from build123d import *

# Parameters (mm, degrees)
ESTRUSIONE_ESTRUSIONE1_DEPTH = 17
SCHIZZO2_W                   = 25
SCHIZZO2_H                   = 30
TAGLIO_ESTRUSIONE1_DEPTH     = 17


with BuildPart() as part:
    # Schizzo1 → Estrusione-Estrusione1 (new body)
    with BuildSketch(Plane.XY):
        with BuildLine():
            Line((0, 0), (85, 0))
            Line((85, 0), (85, 25))
            ThreePointArc((85, 25), (83.753843891, 36.016505892), (80.078350515, 46.47628866))
            Line((80.078350515, 46.47628866), (30, 150))
            Line((30, 150), (0, 150))
            Line((0, 150), (0, 0))
        make_face()
    extrude(amount=ESTRUSIONE_ESTRUSIONE1_DEPTH)

    # Schizzo2 → Taglio-Estrusione1 (cut)
    with BuildSketch(Plane(origin=(0, 0, 0), x_dir=(-1, 0, 0), z_dir=(0, 0, -1))):
        with Locations((-12.5, 15)):
            Rectangle(SCHIZZO2_W, SCHIZZO2_H)
    extrude(amount=-TAGLIO_ESTRUSIONE1_DEPTH, mode=Mode.SUBTRACT)


solid = part.part
Can you work these out from the model? Positions are in its coordinate system, mm. A direction names the side the tool comes from. Give positions to 0.01 mm unless a question says otherwise; leave off trailing zeros. Order: outer loops, then holes, each group sorted by start corner. A loop starts at its lowest first (then second) coordinate and runs counter-clockwise, first axis right, second up. Notation, with made-up numbers: M -5.75,66.5 L 3.25,66.5 A36 cw 3.25,104.5 Z; hole C -16.5,59.5 d2. An arc over 180 degrees is marked long. Use a Markdown table: item, result. Add a question column.
Item 1: Suppose I cut it at A-A (z = 7). List the corners of the cut face in (x, y) for me.
Item 2: For faces 1 (the flat face through (55, 0, 8)), 2 (the flat face through (13, 30, 8)), which set-ups out of +Z, -Z, +X, -X, +Y, -Y let a thin tool reach every point of the face, with its end or its side?
Item 3: If I drill on L1, parallel to X at y = 21, z = 5.25; L2, parallel to Y at x = 14, z = 11; L3, parallel to X at y = 47, z = 5.5, over which ranges is the centre line in solid material (lowest first)? Write a range as [from, to].
Item 4: Suppose I cut it at B-B (x = 18). List the corners of the cut face in (y, z) for me.
Item 5: We'd pull the mould along X, two halves only. Please class faces 3 (the flat face through (0, 91, 8)), 4 (the flat face through (55.39, 97.51, 8.38)), 5 (the flat face through (15, 150, 8)): +X half, -X half, draft (parallel to the pull), parting line (faces both ways), or undercut.
Item 6: Will this pin go through, and if not, where does the flat tip stop? pin 1 (8.5 mm diameter, centred on y = 13, z = 8, fed in from -X).
Item 7: Suppose I cut it at C-C (y = 127). List the corners of the cut face in (x, z) for me, then the cut area to 3 significant figures.
Answer sheet:
| question | item | result |
|---|---|---|
| 1 | outline | M 0,30 L 25,30 L 25,0 L 85,0 L 85,25 A49.32 ccw 80.08,46.48 L 30,150 L 0,150 Z |
| 2 | face 1 | +Z, -Z, +X, -X, -Y |
| 2 | face 2 | +Z, -Z, -X, -Y |
| 3 | L1 | x = [25, 85] |
| 3 | L2 | y = [30, 150] |
| 3 | L3 | x = [0, 79.83] |
| 4 | outline | M 30,0 L 150,0 L 150,17 L 30,17 Z |
| 5 | face 3 | -X half |
| 5 | face 4 | +X half |
| 5 | face 5 | draft |
| 6 | pin 1 | stops at x = 25 |
| 7 | outline | M 0,0 L 41.13,0 L 41.13,17 L 0,17 Z |
| 7 | area | 699 mm² |
